Verification items for this drawing (mm, ordinates from the low corner). Round coordinates to 2 decimals unless told otherwise and drop trailing zeros. Order: outer loops, then holes, each group sorted by start corner. A loop starts at its lowest first (then second) coordinate and runs counter-clockwise, first axis right, second up. Notation, with made-up numbers: M 56.25,26.25 L 90.25,26.25 A21 cw 90.25,38.25 Z; hole C 81,15.5 d5. An arc over 180 degrees is marked long. Return JSON: item names as keys, results as strings. Group by question number.
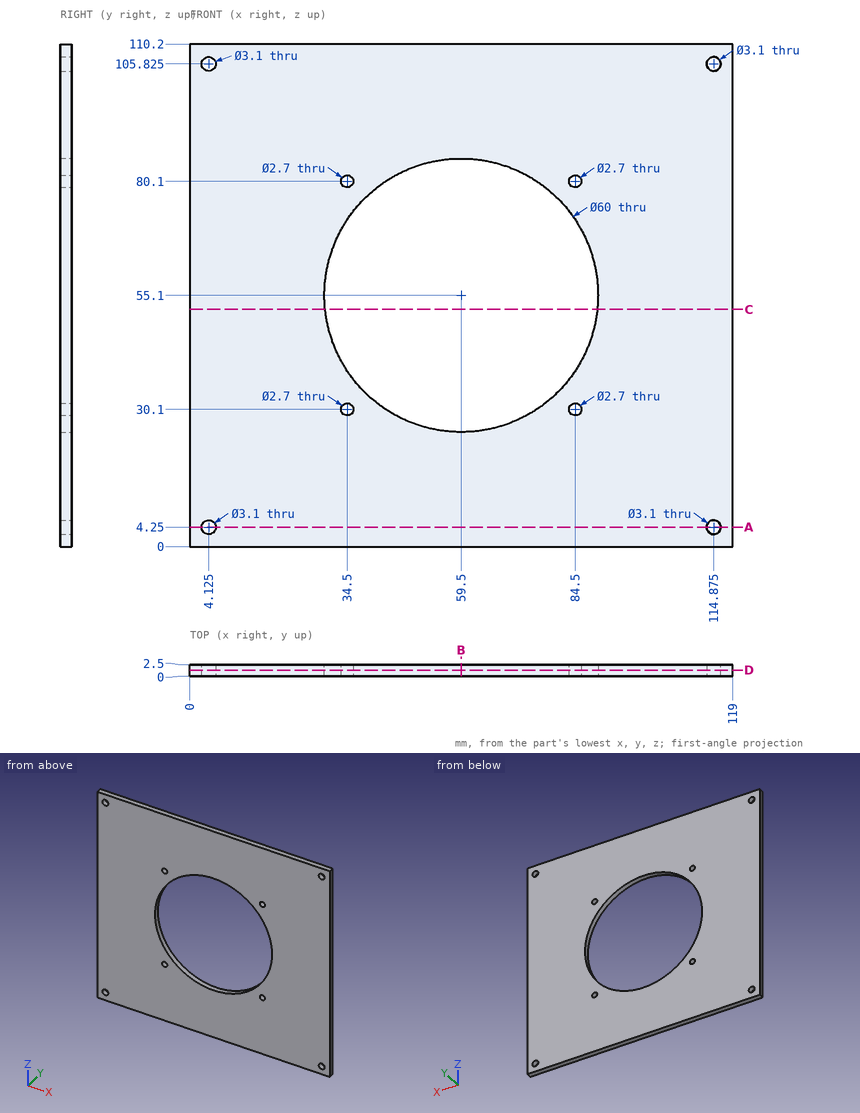
Q1. Section check A-A on z = 4.25. Record the cut outline in (x, y) (3 decimals).
Q2. Section check C-C on z = 52. Record the cut outline in (x, y), plus the area to 3 significant figures.
Q3. Material ranges on line 1 along X through (y, z) = (1.45, 4.25) (3 decimals); line 2 along Z through (x, y) = (59.5, 1.55); line 3 along Z through (x, y) = (34.5, 0.8), recorded low to high.
Q4. Depth check by flat-ended pin: pin 1 Ø2 at (x, z) = (84.5, 80.1) entering from -Y. Enter the tip coordinate at first touch or a pass-through.
Q5. Section check D-D on y = 1.3. Count the separate pieces of the cut face and the enclosed holes in it, plus the area to 3 significant figures.
Q6. Section check B-B on x = 59.5. Record the cut outline in (y, z).
Geometry check:
{
 "1": {"outline": "M 0,0 L 2.575,0 L 2.575,2.5 L 0,2.5 Z; M 5.675,0 L 113.325,0 L 113.325,2.5 L 5.675,2.5 Z; M 116.425,0 L 119,0 L 119,2.5 L 116.425,2.5 Z"},
 "2": {"outline": "M 0,0 L 29.66,0 L 29.66,2.5 L 0,2.5 Z; M 89.34,0 L 119,0 L 119,2.5 L 89.34,2.5 Z", "area": "148 mm^2"},
 "3": {"line 1": "x = 0 to 2.575, 5.675 to 113.325, 116.425 to 119", "line 2": "z = 0 to 25.1, 85.1 to 110.2", "line 3": "z = 0 to 28.75, 31.45 to 38.52, 71.68 to 78.75, 81.45 to 110.2"},
 "4": {"pin 1": "passes through"},
 "5": {"separate pieces": "1", "enclosed holes": "9", "area": "10,200 mm^2"},
 "6": {"outline": "M 0,0 L 2.5,0 L 2.5,25.1 L 0,25.1 Z; M 0,85.1 L 2.5,85.1 L 2.5,110.2 L 0,110.2 Z"}
}
